Print and shaded views of the part. All mm, measured from the part's lowest x, y and z. A direction names the side the tool comes from. Give positions to 0.01 mm unless a question says otherwise; leave off trailing zeros. Loops run counter-clockwise (first coordinate to the right, second up) from the corner with the lowest first, then second, coordinate; pieces in that order, holes last. Notation, with made-up numbers: M 4.5,87 L 51.5,87 A23 ccw 51.5,99 Z; hole C 15,-1 d6. An arc over 180 degrees is marked long. Answer as CSV lines item,"result".
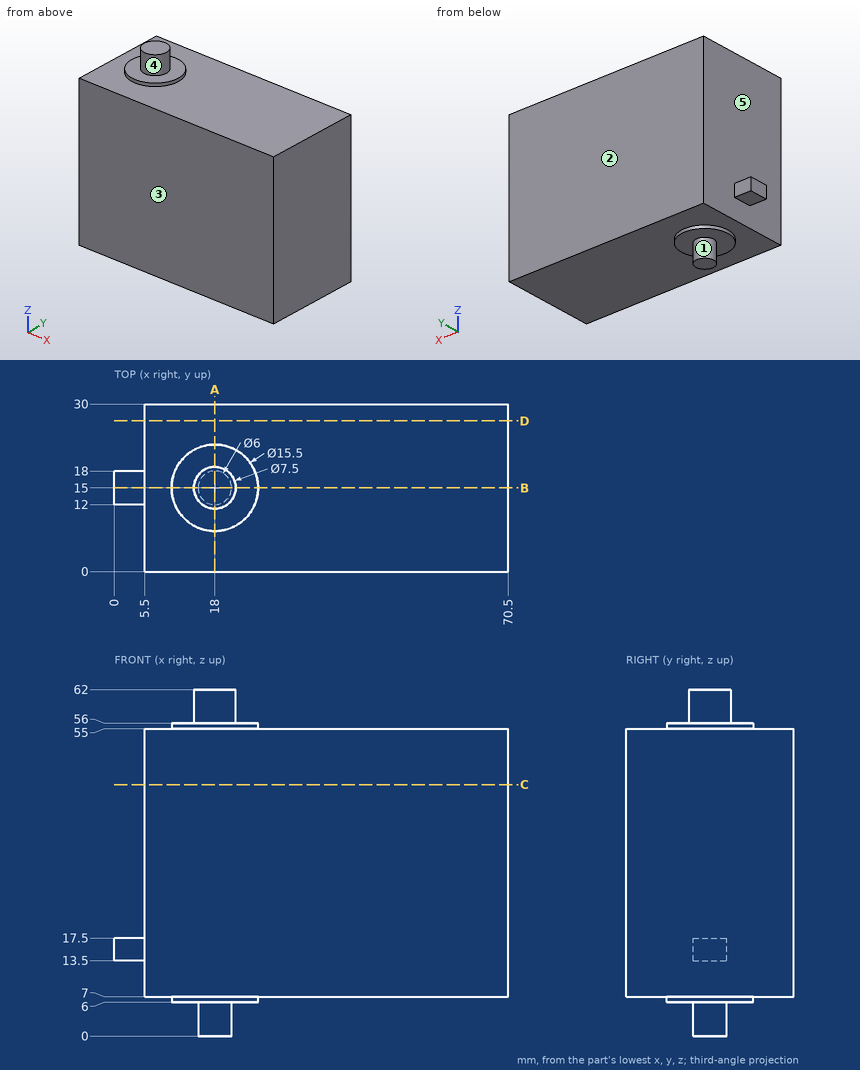
Q1. Which spindle directions (+Z, -Z, +X, -X, +Y, -Y) get a long thin tool onto all of the face, cutting with end or side? Do the marked faces 1 and 2. Say none if no direction does.
Solution:
face 1,"-Z"
face 2,"+Z, -Z, +X, -X, +Y"
Q2. Pin check, flat tips, straight feed: P1, Ø3, axis at x = 2, y = 15.5, coming from the +Z side; P2, Ø10, axis at y = 7, z = 26, coming from the -X side; P3, Ø1.2, axis at x = 3.5, z = 15, coming from the +Y side; P4, Ø5, axis at x = 59.5, z = 25.5, coming from the -Y side. Stop position of each tip, or through.
Solution:
P1,"stops at z = 17.5"
P2,"stops at x = 5.5"
P3,"stops at y = 18"
P4,"stops at y = 0"
Q3. Mould opens along Y. For the marked faces 3, 4 and 5 say: released by +Y, released by -Y, zero draft, split by the parting line, or undercut.
Solution:
face 3,"released by -Y"
face 4,"split by the parting line"
face 5,"zero draft"
Q4. Wall check: line 1 (Z direction, x = 49.5, y = 20); line 2 (X direction, y = 25.75, z = 25.5); line 3 (Z direction, x = 14, y = 12.25). Give the ranges that are in metal, low to high. Write a range as [from, to].
Solution:
line 1,"z = [7, 55]"
line 2,"x = [5.5, 70.5]"
line 3,"z = [6, 56]"
Q5. Cut at D-D (y = 27). Write the cut outline in (x, z).
Solution:
outline,"M 5.5,7 L 70.5,7 L 70.5,55 L 5.5,55 Z"
Q6. Cut at B-B (y = 15). Write the cut outline in (x, z), and give its area (3 significant figures).
Solution:
outline,"M 0,13.5 L 5.5,13.5 L 5.5,7 L 10.25,7 L 10.25,6 L 15,6 L 15,0 L 21,0 L 21,6 L 25.75,6 L 25.75,7 L 70.5,7 L 70.5,55 L 25.75,55 L 25.75,56 L 21.75,56 L 21.75,62 L 14.25,62 L 14.25,56 L 10.25,56 L 10.25,55 L 5.5,55 L 5.5,17.5 L 0,17.5 Z"
area,"3,250 mm²"
Q7. Cut at A-A (x = 18). Write the cut outline in (y, z).
Solution:
outline,"M 0,7 L 7.25,7 L 7.25,6 L 12,6 L 12,0 L 18,0 L 18,6 L 22.75,6 L 22.75,7 L 30,7 L 30,55 L 22.75,55 L 22.75,56 L 18.75,56 L 18.75,62 L 11.25,62 L 11.25,56 L 7.25,56 L 7.25,55 L 0,55 Z"
Q8. Cut at C-C (z = 45). Write the cut outline in (x, y), and give its area (3 significant figures).
Solution:
outline,"M 5.5,0 L 70.5,0 L 70.5,30 L 5.5,30 Z"
area,"1,950 mm²"
